```python
from build123d import *

# Parameters (mm, degrees)
SKETCH1_W           = 5.5
SKETCH1_H           = 39.3
BOSS_EXTRUDE1_DEPTH = 1
CUT_EXTRUDE2_DEPTH  = 1


with BuildPart() as part:
    # Sketch1 → Boss-Extrude1 (new body)
    with BuildSketch(Plane.XY):
        Rectangle(SKETCH1_W, SKETCH1_H)
    extrude(amount=BOSS_EXTRUDE1_DEPTH)

    # Sketch2 → Cut-Extrude2 (cut)
    with BuildSketch(Plane.XY.offset(1)):
        with BuildLine():
            ThreePointArc((-0.25, 12.9), (-1.75, 14.4), (-0.25, 15.9))
            Line((-0.25, 15.9), (-2.75, 15.9))
            Line((-2.75, 15.9), (-2.75, 12.9))
            Line((-2.75, 12.9), (-0.25, 12.9))
        make_face()
        with BuildLine():
            ThreePointArc((1.25, 14.4), (0.810660172, 15.460660172), (-0.25, 15.9))
            Line((-0.25, 15.9), (-0.25, 12.9))
            ThreePointArc((-0.25, 12.9), (0.810660172, 13.339339828), (1.25, 14.4))
        make_face()
        with BuildLine():
            Line((-0.25, 12.9), (-0.25, 15.9))
            ThreePointArc((-0.25, 15.9), (-1.75, 14.4), (-0.25, 12.9))
        make_face()
        with BuildLine():
            Line((-0.25, 9.9), (-2.75, 9.9))
            Line((-2.75, 9.9), (-2.75, 6.9))
            Line((-2.75, 6.9), (-0.25, 6.9))
            ThreePointArc((-0.25, 6.9), (-1.75, 8.4), (-0.25, 9.9))
        make_face()
        with BuildLine():
            ThreePointArc((1.25, 8.4), (0.810660172, 9.460660172), (-0.25, 9.9))
            Line((-0.25, 9.9), (-0.25, 6.9))
            ThreePointArc((-0.25, 6.9), (0.810660172, 7.339339828), (1.25, 8.4))
        make_face()
        with BuildLine():
            Line((-0.25, 6.9), (-0.25, 9.9))
            ThreePointArc((-0.25, 9.9), (-1.75, 8.4), (-0.25, 6.9))
        make_face()
    extrude(amount=-CUT_EXTRUDE2_DEPTH, mode=Mode.SUBTRACT)


solid = part.part
```
Read the model definition and answer for the solid it produces. Units are mm, in the model's axes. A direction names the side the tool comes from. Give positions to 0.01 mm unless a question says otherwise; leave off trailing zeros. Order: outer loops, then holes, each group sorted by start corner. A loop starts at its lowest first (then second) coordinate and runs counter-clockwise, first axis right, second up. Notation, with made-up numbers: (65, 18.25) -> (80, 18.25) arc R19 cw to (80, 45.25) -> close; hole circle Ø2 at (77, -40). An arc over 180 degrees is marked (long way). Write item = value, one per line.
1. Straight lines are drawn through the part: line 1 along Y through (x, z) = (-1.3, 0.5); line 2 along Y through (x, z) = (1, 0.1); line 3 along X through (y, z) = (8.5, 0.1). For each, find the intervals that lie inside material, in ascending order.
Numbers:
line_1 = -19.65 to 6.9, 9.9 to 12.9, 15.9 to 19.65
line_2 = -19.65 to 7.57, 9.23 to 13.57, 15.23 to 19.65
line_3 = 1.25 to 2.75
2. A cutting plane is placed at B-B, the plane z = 0.3. Write down the section's boundary in (x, y), and give its area (3 significant figures).
Numbers:
outline = (-2.75, -19.65) -> (2.75, -19.65) -> (2.75, 19.65) -> (-2.75, 19.65) -> (-2.75, 15.9) -> (-0.25, 15.9) arc R1.5 cw to (-0.25, 12.9) -> (-2.75, 12.9) -> (-2.75, 9.9) -> (-0.25, 9.9) arc R1.5 cw to (-0.25, 6.9) -> (-2.75, 6.9) -> close
area = 194 mm²
3. A cutting plane is placed at A-A, the plane x = -0.9. Write down the section's boundary in (y, z).
Numbers:
outline = (-19.65, 0) -> (6.9, 0) -> (6.9, 1) -> (-19.65, 1) -> close; (9.9, 0) -> (12.9, 0) -> (12.9, 1) -> (9.9, 1) -> close; (15.9, 0) -> (19.65, 0) -> (19.65, 1) -> (15.9, 1) -> close
4. A cutting plane is placed at C-C, the plane y = 15. Write down the section's boundary in (x, z).
Numbers:
outline = (1.12, 0) -> (2.75, 0) -> (2.75, 1) -> (1.12, 1) -> close
5. The mould has two halves that part along Y. Classify faces 1 (the face through (-1.5, 6.9, 0.5)), 2 (the face through (0, 19.65, 0.5)), 3 (the face through (-2.75, -6.6, 0.5)), 4 (the face through (0, -19.65, 0.5)): +Y half, -Y half, draft (parallel to the pull), parting line (faces both ways), or undercut.
Numbers:
face_1 = undercut
face_2 = +Y half
face_3 = draft
face_4 = -Y half
6. For faces 5 (the face through (-2.75, 11.4, 0.5)), 6 (the face through (-1.5, 12.9, 0.5)), determine the directions among +Z, -Z, +X, -X, +Y, -Y from which every point of the face is accessible in a straight line to the end or side of a thin tool.
Numbers:
face_5 = +Z, -Z, -X, +Y, -Y
face_6 = +Z, -Z, -X
